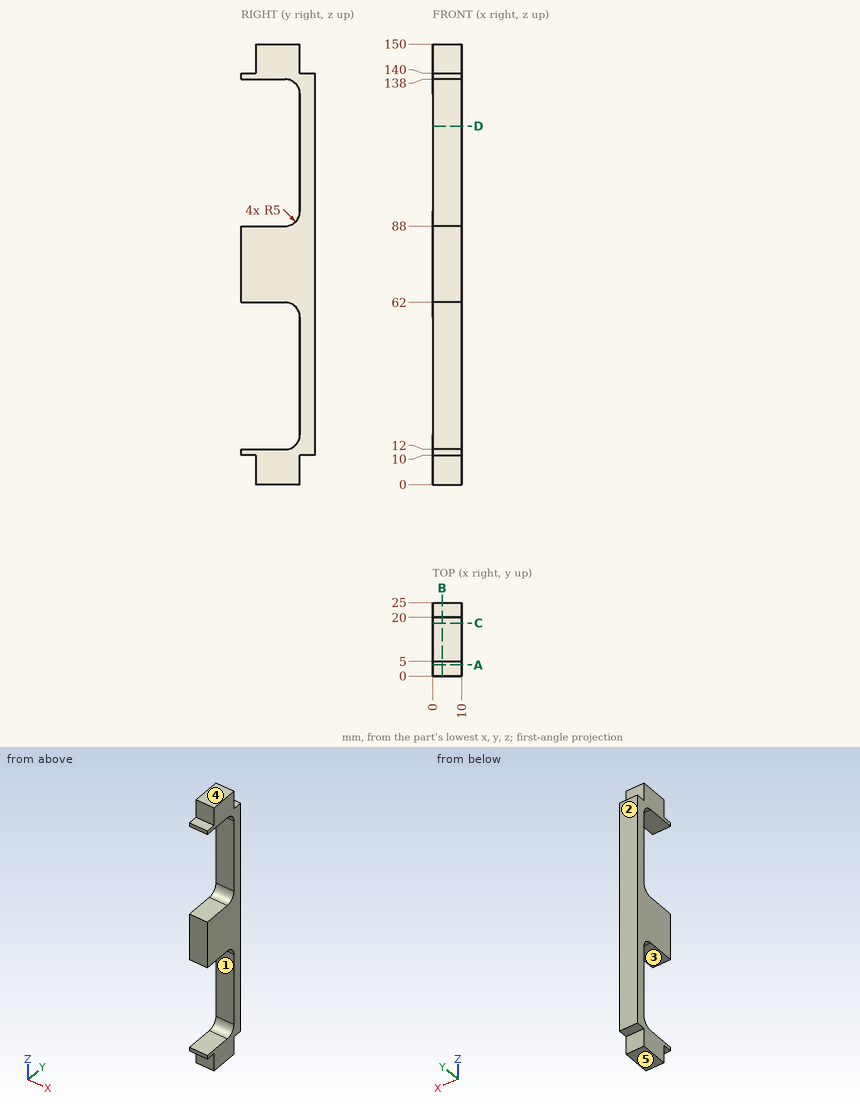
Geometry check sheet. Reference: drawing and pictorial views, mm from the part's lowest x, y, z. A direction names the side the tool comes from. Coordinates: 2 decimals unless noted, no trailing zeros. Order: outer loops, then holes, each group sorted by start corner. A loop starts at its lowest first (then second) coordinate and runs counter-clockwise, first axis right, second up. Notation, with made-up numbers: (-1, 77) -> (27, 77) arc R29 ccw to (27, 102) -> close; hole circle Ø7 at (49, -18.75). An arc over 180 degrees is marked (long way). Use CSV: the item, a comma, the result in double quotes. Start each with the question number.
Q1. Section check C-C, the plane y = 18. Record the cut outline in (x, z).
Q2. Section check D-D, the plane z = 122. Record the cut outline in (x, y).
Q3. Tool access check on the marked faces 1 and 2. Record the directions out of +Z, -Z, +X, -X, +Y, -Y that give a thin tool (end or side, any length) a straight path to the whole face; none if there is none.
Q4. Thickness scan on line 1 along Z through (x, y) = (5, 7.5); line 2 along Z through (x, y) = (2, 20.25); line 3 along Z through (x, y) = (4, 17). Record the ranges inside material, lowest first.
Q5. Draft check along Z on the marked faces 3, 4 and 5. Enter one of: +Z half, -Z half, draft (parallel to the pull), parting line (faces both ways), or undercut.
Q6. Depth check by flat-ended pin: P1, Ø5, axis at x = 4.5, z = 5, coming from the -Y side; P2, Ø2.5, axis at x = 4.5, y = 3, coming from the +Z side; P3, Ø1.5, axis at x = 6.5, y = 3, coming from the -Z side. Enter the tip coordinate at first touch or a pass-through.
Q7. Section check B-B, the plane x = 3.25. Record the cut outline in (y, z), and give its area (3 significant figures).
Q8. Section check A-A, the plane y = 3.75. Record the cut outline in (x, z), and give its area (3 significant figures).
Returned:
1,outline,"(0, 0) -> (10, 0) -> (10, 13) -> (0, 13) -> close; (0, 61) -> (10, 61) -> (10, 89) -> (0, 89) -> close; (0, 137) -> (10, 137) -> (10, 150) -> (0, 150) -> close"
2,outline,"(0, 20) -> (10, 20) -> (10, 25) -> (0, 25) -> close"
3,face 1,"+X, -X, -Y"
3,face 2,"+Z, -Z, +X, -X, +Y"
4,line 1,"z = 0 to 12, 62 to 88, 138 to 150"
4,line 2,"z = 10 to 140"
4,line 3,"z = 0 to 12.42, 61.58 to 88.42, 137.58 to 150"
5,face 3,"undercut"
5,face 4,"+Z half"
5,face 5,"-Z half"
6,P1,"stops at y = 5"
6,P2,"stops at z = 140"
6,P3,"stops at z = 10"
7,outline,"(0, 10) -> (5, 10) -> (5, 0) -> (20, 0) -> (20, 10) -> (25, 10) -> (25, 140) -> (20, 140) -> (20, 150) -> (5, 150) -> (5, 140) -> (0, 140) -> (0, 138) -> (15, 138) arc R5 cw to (20, 133) -> (20, 93) arc R5 cw to (15, 88) -> (0, 88) -> (0, 62) -> (15, 62) arc R5 cw to (20, 57) -> (20, 17) arc R5 cw to (15, 12) -> (0, 12) -> close"
7,area,"1,570 mm^2"
8,outline,"(0, 10) -> (10, 10) -> (10, 12) -> (0, 12) -> close; (0, 62) -> (10, 62) -> (10, 88) -> (0, 88) -> close; (0, 138) -> (10, 138) -> (10, 140) -> (0, 140) -> close"
8,area,"300 mm^2"
